from build123d import *

# Parameters (mm, degrees)
F1_START        = -25.4
F0_R            = 38.1
F1_DEPTH        = 38.1
F2_R            = 6.35
F3_DEPTH        = 50.8
F3_COPIES_COUNT = 5
F4_R            = 38.1
F5_DEPTH        = 35.56
F6_R            = 9.525
F7_DEPTH        = 124.461


# Not quite as in the source:
# - a pattern or mirror of a feature is missing from the dataset's text; its kind, count and spacing are read off the source's solid


with BuildPart() as f1:
    # F0 (on Front) → F1 (new body)
    with BuildSketch(Plane.XZ.offset(F1_START)):
        Circle(F0_R)
    extrude(amount=-F1_DEPTH)

    # F2 (on face) → F3 (join)
    with BuildSketch(Plane.XZ.offset(-25.4)):
        with Locations((0, 25.4)):
            Circle(F2_R)
    f3 = extrude(amount=F3_DEPTH)

    # F3_copies: F3 ×5 about axis
    f3_copies_axis = Axis((0, 0, 0), (0, 1, 0))
    for i in range(1, F3_COPIES_COUNT):
        add(f3.rotate(f3_copies_axis, i * 360 / F3_COPIES_COUNT))

    # F4 (on face) → F5 (join)
    with BuildSketch(Plane.XZ.offset(25.4)):
        Circle(F4_R)
    extrude(amount=F5_DEPTH)

    # F6 (on face) → F7 (cut, through all)
    with BuildSketch(Plane.XZ.offset(60.96)):
        Circle(F6_R)
    extrude(amount=-F7_DEPTH, mode=Mode.SUBTRACT)


solid = f1.part
Could you check a few things on this model? Use its own coordinates, in mm. A direction names the side the tool comes from. Round coordinates to 2 decimals unless told otherwise and drop trailing zeros. Order: outer loops, then holes, each group sorted by start corner. A loop starts at its lowest first (then second) coordinate and runs counter-clockwise, first axis right, second up. Notation, with made-up numbers: M 54,51 L 79,51 A20 cw 79,69 Z; hole C 45.5,-24.75 d5. An arc over 180 degrees is marked long. One line per item, written item: value.
(1) Imagine slicing it at A-A (z = 0). Write out the boundary of the cut face in (x, y) (3 decimals), and give its area (3 significant figures).
Ans:
outline: M -38.1,-60.96 L -9.525,-60.96 L -9.525,-25.4 L -38.1,-25.4 Z; M -38.1,25.4 L -9.525,25.4 L -9.525,63.5 L -38.1,63.5 Z; M 9.525,-60.96 L 38.1,-60.96 L 38.1,-25.4 L 9.525,-25.4 Z; M 9.525,25.4 L 38.1,25.4 L 38.1,63.5 L 9.525,63.5 Z
area: 4,210 mm^2
(2) Imagine slicing it at D-D (z = -12.5). Write out the boundary of the cut face in (x, y), and give its area (3 significant figures).
Ans:
outline: M -35.99,-60.96 L 35.99,-60.96 L 35.99,-25.4 L -35.99,-25.4 Z; M -35.99,25.4 L 35.99,25.4 L 35.99,63.5 L -35.99,63.5 Z
area: 5,300 mm^2
(3) Imagine slicing it at B-B (x = 0). Write out the boundary of the cut face in (y, z) (3 decimals).
Ans:
outline: M -60.96,-38.1 L -25.4,-38.1 L -25.4,-9.525 L -60.96,-9.525 Z; M -60.96,9.525 L -25.4,9.525 L -25.4,19.05 L 25.4,19.05 L 25.4,9.525 L 63.5,9.525 L 63.5,38.1 L 25.4,38.1 L 25.4,31.75 L -25.4,31.75 L -25.4,38.1 L -60.96,38.1 Z; M 25.4,-38.1 L 63.5,-38.1 L 63.5,-9.525 L 25.4,-9.525 Z
(4) Imagine slicing it at C-C (y = 15.5). Write out the boundary of the cut face in (x, z).
Ans:
outline: C -24.16,7.85 d12.7; C -14.93,-20.55 d12.7; C 0,25.4 d12.7; C 14.93,-20.55 d12.7; C 24.16,7.85 d12.7
(5) I need wall thicknesses on line 1 along Y through (x, z) = (-28.5, -23.5); line 2 along Z through (x, y) = (0, 46) (3 decimals); line 3 along X through (y, z) = (-11, -25). Which ranges of each line are inside material? Lowest first, please. Write a range as from..to.
Ans:
line 1: y = -60.96..-25.4, 25.4..63.5
line 2: z = -38.1..-9.525, 9.525..38.1
line 3: x = -19.46..-10.4, 10.4..19.46
(6) I'm going to push flat-ended pins straight in: P1, Ø6, axis at x = 28.5, y = -13.5, coming from the +Z side; P2, Ø4, axis at x = -23.5, y = -30.5, coming from the -Z side; P3, Ø2, axis at y = 19.5, z = 7.5, coming from the -X side. Where does each tip first touch, or does it pass through?
Ans:
P1: stops at z = 14.06
P2: stops at z = -31.45
P3: stops at x = -30.51
(7) Which directions (+Z, -Z, +X, -X, +Y, -Y) give clear straight access to the entire face, cutting with the end or side of a thin tool? Please do faces 4 (the cylindrical face through (-30.235, -42.931, -23.183)), 5 (the cylindrical face through (2.93, 0.356, 19.766)).
Ans:
face 4: +Y, -Y
face 5: none
(8) If we mould it in two halves opening along X, with no side actions, what happens to faces 1 (the cylindrical face through (-30.235, 44.183, -23.183)), 2 (the flat face through (8, -60.96, -8)), 3 (the cylindrical face through (17.836, 0.356, 7.243))? For each: released by +X, released by -X, zero draft, split by the parting line, or undercut.
Ans:
face 1: split by the parting line
face 2: zero draft
face 3: undercut
